Check sheet for the modelled part. Datum: model origin and axes. Units: mm. A direction names the side the tool comes from. Give positions to 0.01 mm unless a question says otherwise; leave off trailing zeros. Write each loop counter-clockwise with the first axis right and the second up, starting at its lowest first coordinate (ties: lowest second). Pieces come first, ordered by that corner, then holes. Notation, with made-up numbers: (88, 56.5) - (100, 56.5) arc R23 cw to (100, 65.5) - close; hole circle Ø2 at (86, 79). An arc over 180 degrees is marked (long way). Return JSON: item names as keys, results as strings. Group by question number.
```python
from build123d import *

# Parameters (mm, degrees)
ESQUISSE1_R                                = 50
BOSS_EXTRU_1_DEPTH                         = 5
ESQUISSE2_R                                = 26
ESQUISSE2_R_2                              = 19
ENL_V_MAT_EXTRU_1_DEPTH                    = 2
ESQUISSE3_R                                = 12.5
ENL_V_MAT_EXTRU_2_DEPTH                    = 71.887234394
CHAMBRAGE_POUR_VIS_T_TE_RONDE_BOMB_2_COUNT = 2
CHAMBRAGE_POUR_VIS_T_TE_RONDE_BOMB_2_PITCH = 49.497474683
CHAMBRAGE_POUR_VIS_T_TE_RONDE_BOMB_3_COUNT = 2
CHAMBRAGE_POUR_VIS_T_TE_RONDE_BOMB_3_PITCH = 70
CHAMBRAGE_POUR_VIS_T_TE_RONDE_BOMB_4_COUNT = 2
CHAMBRAGE_POUR_VIS_T_TE_RONDE_BOMB_4_PITCH = 49.497474683
D_GAGEMENT_M62_D                           = 6.6


with BuildPart() as part:
    # Esquisse1 → Boss.-Extru.1 (new body)
    with BuildSketch(Plane.XY):
        Circle(ESQUISSE1_R)
    extrude(amount=BOSS_EXTRU_1_DEPTH)

    # Esquisse2 → Enlèv. mat.-Extru.1 (cut)
    with BuildSketch(Plane.XY.offset(5)):
        Circle(ESQUISSE2_R)
        Circle(ESQUISSE2_R_2, mode=Mode.SUBTRACT)
    extrude(amount=-ENL_V_MAT_EXTRU_1_DEPTH, mode=Mode.SUBTRACT)

    # Esquisse3 → Enlèv. mat.-Extru.2 (cut, through all)
    with BuildSketch(Plane.XY.offset(5)):
        Circle(ESQUISSE3_R)
    extrude(amount=-ENL_V_MAT_EXTRU_2_DEPTH, mode=Mode.SUBTRACT)

    # Esquisse5 → Chambrage pour vis à tête ronde bombée M41 (revolve, cut)
    with BuildSketch(Plane(origin=(0, 35, 0), x_dir=(0, 1, 0), z_dir=(1, 0, 0))):
        Polygon((0, 0), (0, 5), (2.25, 5), (2.25, 3.125), (2.275, 3.1), (4.5, 3.1), (4.5, 0), align=None)
    chambrage_pour_vis_t_te_ronde_bomb_e_m = revolve(axis=Axis((0, 35, -6.35), (0, 0, 1)), mode=Mode.SUBTRACT)

    # Chambrage pour vis _ t_te ronde bomb 2: Chambrage pour vis à tête ronde bombée M41 ×2
    with Locations(*[Vector(-0.7071067811865476, -0.7071067811865476, 0) * (i * CHAMBRAGE_POUR_VIS_T_TE_RONDE_BOMB_2_PITCH) for i in range(1, CHAMBRAGE_POUR_VIS_T_TE_RONDE_BOMB_2_COUNT)]):
        add(chambrage_pour_vis_t_te_ronde_bomb_e_m, mode=Mode.SUBTRACT)

    # Chambrage pour vis _ t_te ronde bomb 3: Chambrage pour vis à tête ronde bombée M41 ×2
    with Locations(*[(0, -i * CHAMBRAGE_POUR_VIS_T_TE_RONDE_BOMB_3_PITCH, 0) for i in range(1, CHAMBRAGE_POUR_VIS_T_TE_RONDE_BOMB_3_COUNT)]):
        add(chambrage_pour_vis_t_te_ronde_bomb_e_m, mode=Mode.SUBTRACT)

    # Chambrage pour vis _ t_te ronde bomb 4: Chambrage pour vis à tête ronde bombée M41 ×2
    with Locations(*[Vector(0.7071067811865476, -0.7071067811865476, 0) * (i * CHAMBRAGE_POUR_VIS_T_TE_RONDE_BOMB_4_PITCH) for i in range(1, CHAMBRAGE_POUR_VIS_T_TE_RONDE_BOMB_4_COUNT)]):
        add(chambrage_pour_vis_t_te_ronde_bomb_e_m, mode=Mode.SUBTRACT)

    # Dégagement M62 (through all)
    with Locations(Plane.XY.offset(5)):
        with Locations((30.452660491, 27.824413184), (-27.824413184, 30.452660491), (-30.452660491, -27.824413184), (27.824413184, -30.452660491)):
            Hole(D_GAGEMENT_M62_D / 2)


solid = part.part
```
Item 1: Access from +Z, -Z, +X, -X, +Y, -Y to the whole of each face (thin tool, end or side, straight path). Record for faces 1 (the face through (-20.633, -15.821, 4.014)), 2 (the face through (0.86, -32.92, 4.05)), 3 (the face through (37, -2, 3.1)).
Item 2: Section check A-A on z = 1.45. Count the separate pieces of the cut face and the enclosed holes in it, plus the area to 3 significant figures.
Item 3: Depth check by flat-ended pin: pin 1 (2.5 mm diameter, centred on x = 33, y = -2, fed in from -Z); pin 2 (1.5 mm diameter, centred on y = -11, z = 0.5, fed in from -X); pin 3 (1.5 mm diameter, centred on x = 3, z = 2.5, fed in from -Y); pin 4 (4 mm diameter, centred on x = 0, y = -35, fed in from +Z). Enter the tip coordinate at first touch or a pass-through.
Item 4: Material ranges on line 1 along Y through (x, z) = (0, 4.6); line 2 along X through (y, z) = (-0.5, 1.8); line 3 along Y through (x, z) = (14, 3.25), recorded low to high. Write a range as from..to.
Item 5: Mould release check, pull along X, two halves, no side actions. Record for faces 4 (the face through (12.4, -4, 5)), 5 (the face through (47.69, 15.02, 2.46)), 6 (the face through (2, 33, 3.1)): +X half, -X half, draft (parallel to the pull), parting line (faces both ways), or undercut.
Item 6: Section check B-B on x = -35. Record the cut outline in (y, z) (3 decimals).
Reply:
{
 "1": {"face 1": "+Z", "face 2": "+Z, -Z", "face 3": "-Z"},
 "2": {"separate pieces": "1", "enclosed holes": "9", "area": "6,970 mm²"},
 "3": {"pin 1": "z = 3.1", "pin 2": "x = -48.94", "pin 3": "y = -49.95", "pin 4": "through"},
 "4": {"line 1": "-50..-37.25, -32.75..-26, -19..-12.5, 12.5..19, 26..32.75, 37.25..50", "line 2": "-50..-39.47, -30.53..-12.49, 12.49..30.53, 39.47..50", "line 3": "-48..-21.91, -12.85..12.85, 21.91..48"},
 "5": {"face 4": "draft", "face 5": "parting line", "face 6": "undercut"},
 "6": {"outline": "(-35.707, 0) - (-4.5, 0) - (-4.5, 3.1) - (-2.275, 3.1) - (-2.25, 3.125) - (-2.25, 5) - (-35.707, 5) - close; (2.25, 3.125) - (2.275, 3.1) - (4.5, 3.1) - (4.5, 0) - (35.707, 0) - (35.707, 5) - (2.25, 5) - close"}
}
